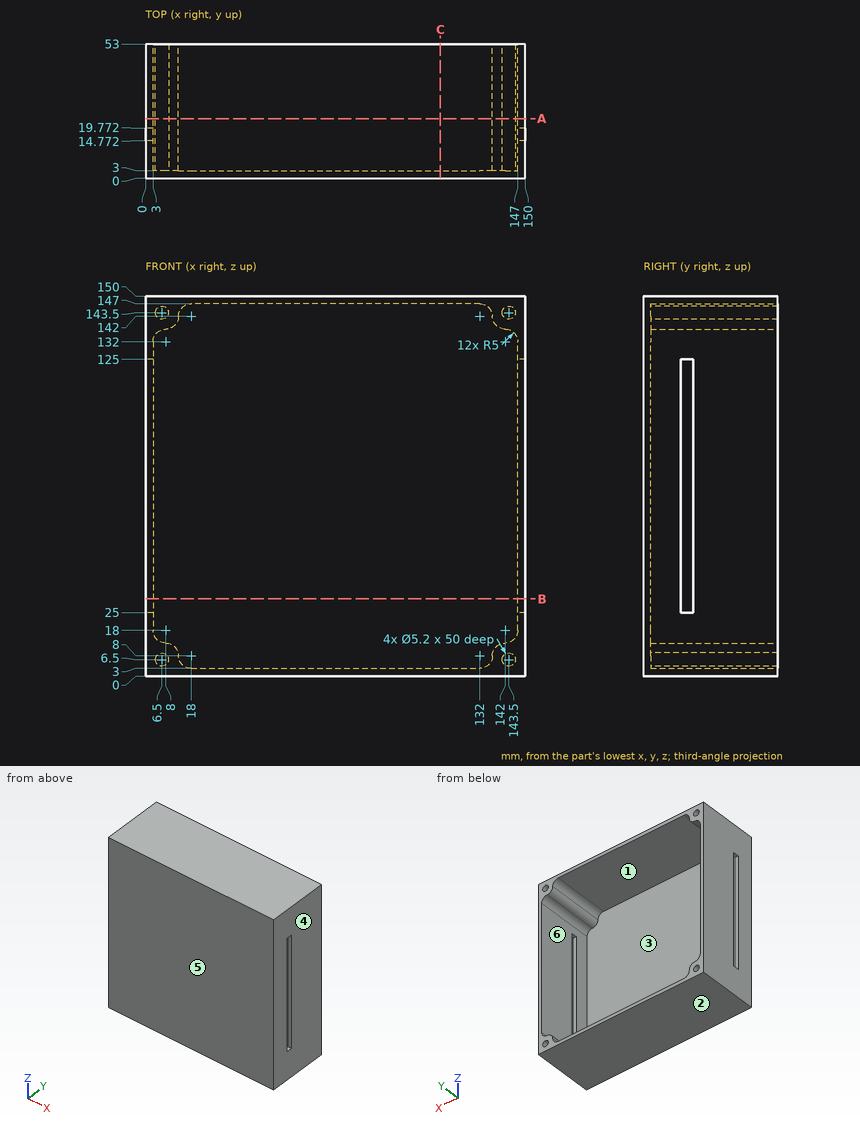
Check sheet for the drawn part. Datum: minimum x, y, z corner. Units: mm. A direction names the side the tool comes from. Round coordinates to 2 decimals unless told otherwise and drop trailing zeros. Loops run counter-clockwise (first coordinate to the right, second up) from the corner with the lowest first, then second, coordinate; pieces in that order, holes last. Notation, with made-up numbers: (51.25, 29) -> (69.25, 29) arc R15 cw to (69.25, 48) -> close; hole circle Ø11 at (-23, 69). An arc over 180 degrees is marked (long way). Put each result on its own line as item: value. Start each with the question number.
1. Section check C-C (x = 116.5). Enter the section's corners in (y, z), plus the area to 3 significant figures.
2. Scan lines: probe 1 along Z at (x, y) = (74.5, 16); probe 2 along X at (y, z) = (20.5, 143.5). Record each from-to range of solid material in increasing order.
3. Gauge pin test, flat ends, axial feed: pin 1 (2.5 mm diameter, centred on x = 1.5, y = 17.5, fed in from -Z); pin 2 (1.6 mm diameter, centred on x = 7, z = 143, fed in from +Y). Record the tip position at first contact, or that the pin passes through.
4. Draft check along Z on the marked faces 1, 2, 3 and 4. Enter one of: +Z half, -Z half, draft (parallel to the pull), parting line (faces both ways), or undercut.
5. Section check A-A (y = 23.5). Enter the section's corners in (x, z), plus the area to 3 significant figures.
6. Access from +Z, -Z, +X, -X, +Y, -Y to the whole of each face (thin tool, end or side, straight path). Record for the marked faces 5 and 6.
7. Section check B-B (z = 30.5). Enter the section's corners in (x, y).
Findings:
1. outline: (0, 0) -> (53, 0) -> (53, 3) -> (3, 3) -> (3, 147) -> (53, 147) -> (53, 150) -> (0, 150) -> close
1. area: 750 mm^2
2. probe 1: z = 0 to 3, 147 to 150
2. probe 2: x = 0 to 3.9, 9.1 to 13.23, 136.77 to 140.9, 146.1 to 150
3. pin 1: stops at z = 0
3. pin 2: stops at y = 3
4. face 1: undercut
4. face 2: -Z half
4. face 3: undercut
4. face 4: draft
5. outline: (0, 0) -> (150, 0) -> (150, 150) -> (0, 150) -> close; hole (3, 18) arc R5 ccw to (8, 13) arc R5 cw to (13, 8) arc R5 ccw to (18, 3) -> (132, 3) arc R5 ccw to (137, 8) arc R5 cw to (142, 13) arc R5 ccw to (147, 18) -> (147, 132) arc R5 ccw to (142, 137) arc R5 cw to (137, 142) arc R5 ccw to (132, 147) -> (18, 147) arc R5 ccw to (13, 142) arc R5 cw to (8, 137) arc R5 ccw to (3, 132) -> close; hole circle Ø5.2 at (6.5, 6.5); hole circle Ø5.2 at (6.5, 143.5); hole circle Ø5.2 at (143.5, 6.5); hole circle Ø5.2 at (143.5, 143.5)
5. area: 2,100 mm^2
6. face 5: +Z, -Z, +X, -X, -Y
6. face 6: +Y
7. outline: (0, 0) -> (150, 0) -> (150, 14.77) -> (147, 14.77) -> (147, 3) -> (3, 3) -> (3, 14.77) -> (0, 14.77) -> close; (0, 19.77) -> (3, 19.77) -> (3, 53) -> (0, 53) -> close; (147, 19.77) -> (150, 19.77) -> (150, 53) -> (147, 53) -> close
